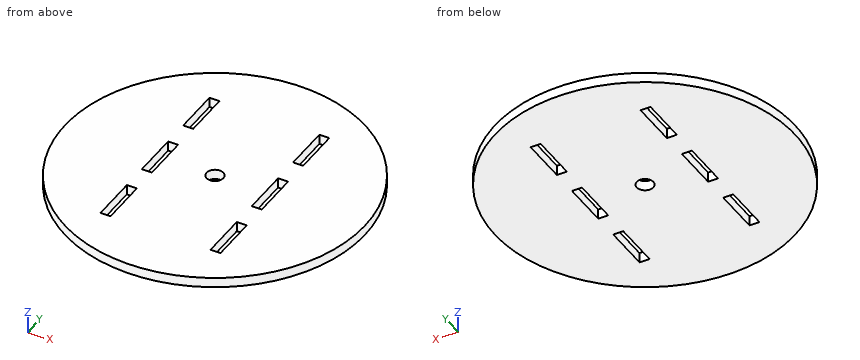
```python
from build123d import *

# Parameters (mm, degrees)
SKETCH1_R           = 45
BOSS_EXTRUDE1_DEPTH = 3
SKETCH2_R           = 2.5
SKETCH2_W           = 3
SKETCH2_H           = 14
CUT_EXTRUDE3_DEPTH  = 35


with BuildPart() as part:
    # Sketch1 → Boss-Extrude1 (new body)
    with BuildSketch(Plane.XY):
        with Locations((45, 147.5080997)):
            Circle(SKETCH1_R)
    extrude(amount=BOSS_EXTRUDE1_DEPTH)

    # Sketch2 → Cut-Extrude3 (cut)
    with BuildSketch(Plane.XY):
        with Locations((45, 147.5080997)):
            Circle(SKETCH2_R)
        with Locations((61.5, 169.5080997)):
            Rectangle(SKETCH2_W, SKETCH2_H)
        with Locations((61.5, 147.5080997)):
            Rectangle(SKETCH2_W, SKETCH2_H)
        with Locations((61.5, 125.5080997)):
            Rectangle(SKETCH2_W, SKETCH2_H)
        with Locations((28.5, 169.5080997)):
            Rectangle(SKETCH2_W, SKETCH2_H)
        with Locations((28.5, 125.5080997)):
            Rectangle(SKETCH2_W, SKETCH2_H)
        with Locations((28.5, 147.5080997)):
            Rectangle(SKETCH2_W, SKETCH2_H)
    extrude(amount=CUT_EXTRUDE3_DEPTH, mode=Mode.SUBTRACT)


solid = part.part
```
Read the model definition and answer for the solid it produces. Units are mm, in the model's axes. Give positions to 0.01 mm unless a question says otherwise; leave off trailing zeros. Order: outer loops, then holes, each group sorted by start corner. A loop starts at its lowest first (then second) coordinate and runs counter-clockwise, first axis right, second up.
(1) Straight lines are drawn through the part: L1, parallel to X at y = 147.5, z = 0.55; L2, parallel to Y at x = 45, z = 1.8; L3, parallel to X at y = 120.5, z = 0.2. For each, find the intervals that lie inside material, in ascending order.
(2) Find section B-B (y = 130.5). Give the vertices of the cut face in (x, z), plus the area to 3 significant figures.
(3) Find section C-C (z = 2.4). Give the vertices of the cut face in (x, y), plus the area to 3 significant figures.
(4) Find section D-D (y = 152). Give the vertices of the cut face in (x, z), plus the area to 3 significant figures.
(5) Find section A-A (x = 45). Give the vertices of the cut face in (y, z), plus the area to 3 significant figures.
(6) Given pin 1 (1.5 mm diameter, centred on y = 124, z = 1, fed in from +X); pin 2 (2 mm diameter, centred on x = 58.5, y = 141.5, fed in from -Z); pin 3 (0.9 mm diameter, centred on y = 125.5, z = 1, fed in from +X); pin 4 (1 mm diameter, centred on x = 75.5, z = 1.5, fed in from -Y), each flat-ended and moving along its own axis, determine where each tip first touches the part or whether it passes through.
Result sheet:
1. L1: x = 0 to 27, 30 to 42.5, 47.5 to 60, 63 to 90
1. L2: y = 102.51 to 145.01, 150.01 to 192.51
1. L3: x = 9.01 to 27, 30 to 60, 63 to 80.99
2. outline: (3.34, 0) - (27, 0) - (27, 3) - (3.34, 3) - close; (30, 0) - (60, 0) - (60, 3) - (30, 3) - close; (63, 0) - (86.66, 0) - (86.66, 3) - (63, 3) - close
2. area: 232 mm2
3. outline: circle Ø90 at (45, 147.51); hole (27, 118.51) - (30, 118.51) - (30, 132.51) - (27, 132.51) - close; hole (27, 140.51) - (30, 140.51) - (30, 154.51) - (27, 154.51) - close; hole (27, 162.51) - (30, 162.51) - (30, 176.51) - (27, 176.51) - close; hole circle Ø5 at (45, 147.51); hole (60, 118.51) - (63, 118.51) - (63, 132.51) - (60, 132.51) - close; hole (60, 140.51) - (63, 140.51) - (63, 154.51) - (60, 154.51) - close; hole (60, 162.51) - (63, 162.51) - (63, 176.51) - (60, 176.51) - close
3. area: 6,090 mm2
4. outline: (0.22, 0) - (27, 0) - (27, 3) - (0.22, 3) - close; (30, 0) - (60, 0) - (60, 3) - (30, 3) - close; (63, 0) - (89.78, 0) - (89.78, 3) - (63, 3) - close
4. area: 251 mm2
5. outline: (102.51, 0) - (145.01, 0) - (145.01, 3) - (102.51, 3) - close; (150.01, 0) - (192.51, 0) - (192.51, 3) - (150.01, 3) - close
5. area: 255 mm2
6. pin 1: stops at x = 83.82
6. pin 2: stops at z = 0
6. pin 3: stops at x = 84.5
6. pin 4: stops at y = 113.97
